Read the model definition and answer for the solid it produces. Units are mm, in the model's axes. Give positions to 0.01 mm unless a question says otherwise; leave off trailing zeros. Order: outer loops, then holes, each group sorted by start corner. A loop starts at its lowest first (then second) coordinate and runs counter-clockwise, first axis right, second up. Notation, with made-up numbers: M 18,33.5 L 32,33.5 A12 cw 32,55.5 Z; hole C 77.5,-0.75 d11. An arc over 180 degrees is marked long. One line per item, written item: value.
Autodesk Inventor part; units mm, degrees
ref_plane "YZ Plane" through (0, 0, 0) normal (1, 0, 0) x (0, 1, 0)
ref_plane "XZ Plane" through (0, 0, 0) normal (0, 1, 0) x (-1, 0, 0)
ref_plane "XY Plane" through (0, 0, 0) normal (0, 0, 1) x (1, 0, 0)
sketch "Sketch1" plane through (0, 0, 0) normal (0, 0, 1) x (1, 0, 0)
  circle A0 centre (0, 0) radius 92.5
  dimension "d22" = 185
extrude "Plate1" add sketch "Sketch1" along normal blind 3
sketch "Sketch5" plane through (0, 0, 3) normal (0, 0, 1) x (1, 0, 0)
  circle A0 centre (0, 0) radius 92.5
  circle A1 centre (0, 72.5) radius 9
  circle A2 centre (0, 0) radius 72.5 construction
  dimension "d23" = 18
  dimension "d30" = 20
extrude "Cut1" cut sketch "Sketch5" against normal blind 3 contours A1
pattern_circular "Circular Pattern1" count 8 over 360 about axis through (0, 0, 0) along (0, 0, 1) of "Cut1"
equation "\"d25\" = Thickness"
equation "\"d2\" = Thickness"
equation "\"BendReliefWidth\" = Thickness"
equation "\"BendReliefDepth\" = 0.5 * Thickness"
equation "\"CornerReliefSize\" = 4 * Thickness"
equation "\"MinimumRemnant\" = 2 * Thickness"
equation "\"TransitionRadius\" = BendRadius"
equation "\"JacobiRadiusSize\" = BendRadius"
equation "\"GapSize\" = Thickness"
properties part number "MSC 921 plug 76" material "Stainless Steel"
1) Find section D-D, the plane z = 0.95. Count the separate pieces of the cut face and the enclosed holes in it, plus the area to 3 significant figures.
Reported:
separate pieces: 1
enclosed holes: 8
area: 24,800 mm^2
2) Find section C-C, the plane x = 72.5. Write down the section's boundary in (y, z), plus the area to 3 significant figures.
Reported:
outline: M -57.45,0 L -9,0 L -9,3 L -57.45,3 Z; M 9,0 L 57.45,0 L 57.45,3 L 9,3 Z
area: 291 mm^2
3) Determine the mould class of faces 1 (the face through (-1, 1, 0)), 2 (the face through (-1, 1, 3)), 3 (the face through (-63.714, -1.951, 1.521)) for opening direction Z: +Z half, -Z half, draft (parallel to the pull), parting line (faces both ways), or undercut.
Reported:
face 1: -Z half
face 2: +Z half
face 3: draft
4) Find section B-B, the plane y = 55.5. Write down the section's boundary in (x, z).
Reported:
outline: M -74,0 L -59.21,0 L -59.21,3 L -74,3 Z; M -43.32,0 L 43.32,0 L 43.32,3 L -43.32,3 Z; M 59.21,0 L 74,0 L 74,3 L 59.21,3 Z
5) Find section A-A, the plane x = 0. Write down the section's boundary in (y, z), plus the area to 3 significant figures.
Reported:
outline: M -92.5,0 L -81.5,0 L -81.5,3 L -92.5,3 Z; M -63.5,0 L 63.5,0 L 63.5,3 L -63.5,3 Z; M 81.5,0 L 92.5,0 L 92.5,3 L 81.5,3 Z
area: 447 mm^2
6) This flat-tipped pin is pushed along its axis until it touches: pin 1 Ø11 at (x, y) = (-51.27, 51.27) entering from -Z. Where does it stop, or does it pass through?
Reported:
pin 1: passes through
7) Consider probe 1 along Y at (x, z) = (0, 2); probe 2 along Y at (x, z) = (-56, 1.1); probe 3 along X at (y, z) = (49, 0.3). Determine where each line is inside the solid, lowest interval first.
Reported:
probe 1: y = -92.5 to -81.5, -63.5 to 63.5, 81.5 to 92.5
probe 2: y = -73.62 to -58.92, -43.61 to 43.61, 58.92 to 73.62
probe 3: x = -78.46 to -59.98, -42.55 to 42.55, 59.98 to 78.46
